Verification items for the finished model (mm, model axes). A direction names the side the tool comes from. Give positions to 0.01 mm unless a question says otherwise; leave off trailing zeros. Order: outer loops, then holes, each group sorted by start corner. A loop starts at its lowest first (then second) coordinate and runs counter-clockwise, first axis right, second up. Notation, with made-up numbers: (62.5, -29.5) -> (74.5, -29.5) arc R19 cw to (74.5, -9.5) -> close; hole circle Ø3 at (-14, 23.5). An arc over 180 degrees is marked (long way). Write each question's results on one line, items separated by ' | '. Start each with the question number.
1. Cross-section at C-C, the plane x = 104. Enter the section's corners in (y, z).
2. Cross-section at B-B, the plane x = 40. Enter the section's corners in (y, z).
3. Material ranges on L1, parallel to X at y = 4.95, z = 163.95; L2, parallel to X at y = 9.75, z = 188; L3, parallel to X at y = 9.6, z = 156.45, recorded low to high. Write a range as from..to.
4. Depth check by flat-ended pin: pin 1 Ø9 at (x, z) = (14, 166) entering from -Y; pin 2 Ø8 at (y, z) = (7, 167) entering from +X; pin 3 Ø9 at (x, z) = (-11.5, 165) entering from -Y; pin 4 Ø1.9 at (x, y) = (62, 8) entering from -Z. Enter the tip coordinate at first touch or a pass-through.
5. Set-up check for faces 4 (the face through (11, 6.8, 181)), 5 (the face through (41.897, 7.131, 148.66)): record each of +Z, -Z, +X, -X, +Y, -Y from which the full face is reachable in a straight line by a thin tool's end or side.
6. Cross-section at A-A, the plane x = 144. Enter the section's corners in (y, z).
7. Mould release check, pull along Z, two halves, no side actions. Record for faces 1 (the face through (84, 7.1, 171.3)), 2 (the face through (65, 7, 180.45)), 3 (the face through (7, -4, 175)): +Z half, -Z half, draft (parallel to the pull), parting line (faces both ways), or undercut.
from build123d import *

# Parameters (mm, degrees)
PLACA_START                     = 4
PLACA_DEPTH                     = 6.35
PLACA_R1_START                  = 4
CROQUIS14_R                     = 35
PLACA_R1_DEPTH                  = 6.35
PLACA_R2_START                  = 4
CROQUIS15_R                     = 30
PLACA_R2_DEPTH                  = 6.35
ALIGERADO_START                 = 4
ALIGERADO_DEPTH                 = 6.35
BARRENOS_SEPARADORES_M4_START   = 4
CROQUIS17_R                     = 2.25
BARRENOS_SEPARADORES_M4_DEPTH   = 6.35
BARRENOS_M2_Y_M3_START          = 4
CROQUIS18_R                     = 2.25
CROQUIS18_R_2                   = 2.6
CROQUIS18_R_3                   = 5.5
CROQUIS18_R_4                   = 18
CROQUIS18_R_5                   = 1.45
BARRENOS_M2_Y_M3_DEPTH          = 6.35
REFRENTADO_M4_CABEZA_BAJA_START = 4
CROQUIS19_R                     = 4
REFRENTADO_M4_CABEZA_BAJA_DEPTH = 2.8
REFRENTADO_M2_5_START           = 4
CROQUIS20_R                     = 2.8
REFRENTADO_M2_5_DEPTH           = 2.6
ROSCA_M3_BASES_CINCHO_START     = 4
CROQUIS21_R                     = 1.25
ROSCA_M3_BASES_CINCHO_DEPTH     = 6.35
PASO_M3_BASES_CINCHO_START      = 4
CROQUIS22_R                     = 1.7
PASO_M3_BASES_CINCHO_DEPTH      = 6.35
CROQUIS23_R                     = 10
SALIENTE_EXTRUIR1_DEPTH         = 8
CROQUIS24_R                     = 7.475
CORTAR_EXTRUIR1_DEPTH           = 5.5


with BuildPart() as part:
    # Croquis13 → Placa (new body)
    with BuildSketch(Plane(origin=(0, 0, 0), x_dir=(1, 0, 0), z_dir=(0, 1, 0)).offset(PLACA_START)):
        Polygon((1.148293963, -206.431158085), (153.384251969, -201.433849787), (153.384251969, -141.466150213), (1.148293963, -136.468841915), align=None)
    extrude(amount=PLACA_DEPTH)

    # Croquis14 → Placa_r1 (add)
    with BuildSketch(Plane(origin=(0, 0, 0), x_dir=(1, 0, 0), z_dir=(0, 1, 0)).offset(PLACA_R1_START)):
        with Locations((0, -171.45)):
            Circle(CROQUIS14_R)
    extrude(amount=PLACA_R1_DEPTH)

    # Croquis15 → Placa_r2 (add)
    with BuildSketch(Plane(origin=(0, 0, 0), x_dir=(1, 0, 0), z_dir=(0, 1, 0)).offset(PLACA_R2_START)):
        with Locations((152.4, -171.45)):
            Circle(CROQUIS15_R)
    extrude(amount=PLACA_R2_DEPTH)

    # Croquis16 → Aligerado (cut)
    with BuildSketch(Plane(origin=(0, 0, 0), x_dir=(1, 0, 0), z_dir=(0, 1, 0)).offset(ALIGERADO_START)):
        with BuildLine():
            Line((55, -162.45), (75, -162.45))
            ThreePointArc((75, -162.45), (84, -171.45), (75, -180.45))
            Line((75, -180.45), (55, -180.45))
            ThreePointArc((55, -180.45), (46, -171.45), (55, -162.45))
        make_face()
    extrude(amount=ALIGERADO_DEPTH, mode=Mode.SUBTRACT)

    # Croquis17 → Barrenos_separadores_M4 (cut)
    with BuildSketch(Plane(origin=(0, 0, 0), x_dir=(1, 0, 0), z_dir=(0, 1, 0)).offset(BARRENOS_SEPARADORES_M4_START)):
        with Locations(Location((40, -195.45, 0), (0, 0, 270))):
            Circle(CROQUIS17_R)
        with Locations(Location((40, -147.45, 0), (0, 0, 270))):
            Circle(CROQUIS17_R)
        with Locations(Location((90, -191.45, 0), (0, 0, 270))):
            Circle(CROQUIS17_R)
        with Locations(Location((90, -151.45, 0), (0, 0, 270))):
            Circle(CROQUIS17_R)
    extrude(amount=BARRENOS_SEPARADORES_M4_DEPTH, mode=Mode.SUBTRACT)

    # Croquis18 → Barrenos_M2_y_M3 (cut)
    with BuildSketch(Plane(origin=(0, 0, 0), x_dir=(1, 0, 0), z_dir=(0, 1, 0)).offset(BARRENOS_M2_Y_M3_START)):
        with Locations(Location((12.990381057, -178.95, 0), (0, 0, 270))):
            Circle(CROQUIS18_R)
        with Locations(Location((0, -186.45, 0), (0, 0, 270))):
            Circle(CROQUIS18_R)
        with Locations(Location((-12.990381057, -178.95, 0), (0, 0, 270))):
            Circle(CROQUIS18_R)
        with Locations(Location((-12.990381057, -163.95, 0), (0, 0, 270))):
            Circle(CROQUIS18_R)
        with Locations(Location((0, -156.45, 0), (0, 0, 270))):
            Circle(CROQUIS18_R)
        with Locations(Location((12.990381057, -163.95, 0), (0, 0, 270))):
            Circle(CROQUIS18_R)
        with Locations(Location((7.125, -183.790862004, 0), (0, 0, 270))):
            Circle(CROQUIS18_R_2)
        with Locations(Location((-14.25, -171.45, 0), (0, 0, 270))):
            Circle(CROQUIS18_R_2)
        with Locations(Location((7.125, -159.109137996, 0), (0, 0, 270))):
            Circle(CROQUIS18_R_2)
        with Locations(Location((0, -171.45, 0), (0, 0, 270))):
            Circle(CROQUIS18_R_3)
        with Locations(Location((152.4, -171.45, 0), (0, 0, 270))):
            Circle(CROQUIS18_R_4)
        with Locations(Location((172.65, -171.45, 0), (0, 0, 270))):
            Circle(CROQUIS18_R_5)
        with Locations(Location((166.718912319, -185.768912319, 0), (0, 0, 270))):
            Circle(CROQUIS18_R_5)
        with Locations(Location((152.4, -191.7, 0), (0, 0, 270))):
            Circle(CROQUIS18_R_5)
        with Locations(Location((138.081087681, -185.768912319, 0), (0, 0, 270))):
            Circle(CROQUIS18_R_5)
        with Locations(Location((132.15, -171.45, 0), (0, 0, 270))):
            Circle(CROQUIS18_R_5)
        with Locations(Location((138.081087681, -157.131087681, 0), (0, 0, 270))):
            Circle(CROQUIS18_R_5)
        with Locations(Location((152.4, -151.2, 0), (0, 0, 270))):
            Circle(CROQUIS18_R_5)
        with Locations(Location((166.718912319, -157.131087681, 0), (0, 0, 270))):
            Circle(CROQUIS18_R_5)
    extrude(amount=BARRENOS_M2_Y_M3_DEPTH, mode=Mode.SUBTRACT)

    # Croquis19 → Refrentado_M4_cabeza_baja (cut)
    with BuildSketch(Plane(origin=(0, 0, 0), x_dir=(1, 0, 0), z_dir=(0, 1, 0)).offset(REFRENTADO_M4_CABEZA_BAJA_START)):
        with Locations(Location((12.990381057, -178.95, 0), (0, 0, 270))):
            Circle(CROQUIS19_R)
        with Locations(Location((0, -186.45, 0), (0, 0, 270))):
            Circle(CROQUIS19_R)
        with Locations(Location((-12.990381057, -178.95, 0), (0, 0, 270))):
            Circle(CROQUIS19_R)
        with Locations(Location((-12.990381057, -163.95, 0), (0, 0, 270))):
            Circle(CROQUIS19_R)
        with Locations(Location((0, -156.45, 0), (0, 0, 270))):
            Circle(CROQUIS19_R)
        with Locations(Location((12.990381057, -163.95, 0), (0, 0, 270))):
            Circle(CROQUIS19_R)
    extrude(amount=REFRENTADO_M4_CABEZA_BAJA_DEPTH, mode=Mode.SUBTRACT)

    # Croquis20 → Refrentado_M2-5 (cut)
    with BuildSketch(Plane(origin=(0, 0, 0), x_dir=(1, 0, 0), z_dir=(0, 1, 0)).offset(REFRENTADO_M2_5_START)):
        with Locations((172.65, -171.45)):
            Circle(CROQUIS20_R)
        with Locations((166.718912319, -185.768912319)):
            Circle(CROQUIS20_R)
        with Locations((152.4, -191.7)):
            Circle(CROQUIS20_R)
        with Locations((138.081087681, -185.768912319)):
            Circle(CROQUIS20_R)
        with Locations((132.15, -171.45)):
            Circle(CROQUIS20_R)
        with Locations((138.081087681, -157.131087681)):
            Circle(CROQUIS20_R)
        with Locations((152.4, -151.2)):
            Circle(CROQUIS20_R)
        with Locations((166.718912319, -157.131087681)):
            Circle(CROQUIS20_R)
    extrude(amount=REFRENTADO_M2_5_DEPTH, mode=Mode.SUBTRACT)

    # Croquis21 → Rosca_M3_bases_cincho (cut)
    with BuildSketch(Plane(origin=(0, 0, 0), x_dir=(1, 0, 0), z_dir=(0, 1, 0)).offset(ROSCA_M3_BASES_CINCHO_START)):
        with Locations(Location((112, -171.45, 0), (0, 0, 270))):
            Circle(CROQUIS21_R)
    extrude(amount=ROSCA_M3_BASES_CINCHO_DEPTH, mode=Mode.SUBTRACT)

    # Croquis22 → Paso_M3_bases_cincho (cut)
    with BuildSketch(Plane(origin=(0, 0, 0), x_dir=(1, 0, 0), z_dir=(0, 1, 0)).offset(PASO_M3_BASES_CINCHO_START)):
        with Locations(Location((112, -171.45, 0), (0, 0, 270))):
            Circle(CROQUIS22_R)
    extrude(amount=PASO_M3_BASES_CINCHO_DEPTH, mode=Mode.SUBTRACT)

    # Croquis23 → Saliente-Extruir1 (add)
    with BuildSketch(Plane.XZ.offset(-4)):
        with Locations(Location((0, 171.45, 0), (0, 0, 90))):
            Circle(CROQUIS23_R)
    extrude(amount=SALIENTE_EXTRUIR1_DEPTH)

    # Croquis24 → Cortar-Extruir1 (cut)
    with BuildSketch(Plane.XZ.offset(4)):
        with Locations(Location((0, 171.45, 0), (0, 0, 270))):
            Circle(CROQUIS24_R)
    extrude(amount=-CORTAR_EXTRUIR1_DEPTH, mode=Mode.SUBTRACT)


solid = part.part
Results below:
1) outline: (4, 139.85) -> (10.35, 139.85) -> (10.35, 203.05) -> (4, 203.05) -> close
2) outline: (4, 137.74) -> (10.35, 137.74) -> (10.35, 145.2) -> (4, 145.2) -> close; (4, 149.7) -> (10.35, 149.7) -> (10.35, 193.2) -> (4, 193.2) -> close; (4, 197.7) -> (10.35, 197.7) -> (10.35, 205.16) -> (4, 205.16) -> close
3) L1: x = -34.19..-16.99, -8.99..8.99, 16.99..50.03, 79.97..136.04, 168.76..181.45 | L2: x = -30.84..-1.63, 1.63..145.32, 159.48..177.42 | L3: x = -31.62..-2.25, 2.25..136.8, 139.36..142.45, 162.35..165.44, 168..178.38
4) pin 1: stops at y = 4 | pin 2: stops at x = 182.4 | pin 3: stops at y = -4 | pin 4: stops at z = 138.44
5) face 4: -Y | face 5: +Y, -Y
6) outline: (4, 141.16) -> (10.35, 141.16) -> (10.35, 155.53) -> (4, 155.53) -> close; (4, 187.37) -> (10.35, 187.37) -> (10.35, 201.74) -> (4, 201.74) -> close
7) face 1: undercut | face 2: undercut | face 3: draft
